Part model, mm, in its own coordinate system. A direction names the side the tool comes from. Round coordinates to 2 decimals unless told otherwise and drop trailing zeros. Write each loop counter-clockwise with the first axis right and the second up, starting at its lowest first coordinate (ties: lowest second). Pieces come first, ordered by that corner, then holes.
1) Saw through at C-C on x = 7. Write the cut outline in (y, z), and give its area (3 significant figures).
2) Saw through at D-D on y = 18.25. Write the cut outline in (x, z), and give its area (3 significant figures).
3) Saw through at A-A on y = 8. Write the cut outline in (x, z), and give its area (3 significant figures).
4) Drill centre lines: L1, parallel to Y at x = 39.5, z = 1; L2, parallel to X at y = 14.5, z = 4; L3, parallel to X at y = 13.75, z = 1.25. Where is each one in solid material? Low to high.
5) Which spindle directions (+Z, -Z, +X, -X, +Y, -Y) get a long thin tool onto all of the face, cutting with end or side? Do faces 1 (the flat face through (37.795, 10, 2)), 2 (the flat face through (47, 5, 8)), 3 (the flat face through (4, 5, 6)). Say none if no direction does.
6) Saw through at B-B on z = 6.5. Write the cut outline in (x, y).
7) Flat gauge pins, fed straight in: pin 1 (10 mm diameter, centred on x = 40.5, y = 6, fed in from +Z); pin 2 (2.5 mm diameter, centred on x = 4, z = 11.5, fed in from +Y); pin 3 (1 mm diameter, centred on x = 29.5, y = 5, fed in from +Z). Where does each tip first touch, or does it go through?
8) Pull direction X, two halves, no side cores. Call faces 4 (the cylindrical face through (16.04, 6.2, 2.54)), 5 (the cylindrical face through (10.69, 6.14, 2.54)), 6 (the flat face through (25, 0, 4)): +X half, -X half, draft (parallel to the pull), parting line (faces both ways), or undercut.
```python
from build123d import *

# Parameters (mm, degrees)
SKETCH1_R           = 8.106403635
SKETCH1_R_2         = 8.1
BOSS_EXTRUDE2_DEPTH = 5
FILLET1_R           = 4
SKETCH3_W           = 5.205268412
SKETCH3_H           = 16.38085221
BOSS_EXTRUDE3_DEPTH = 5
SKETCH2_R           = 1.575419973
CUT_EXTRUDE1_DEPTH  = 5


with BuildPart() as part:
    # Sketch1 → Boss-Extrude2 (new body)
    with BuildSketch(Plane.XY):
        with BuildLine():
            Line((0, 0), (50, 0))
            Line((50, 0), (50, 5))
            Line((50, 5), (40.794731588, 5))
            Line((40.794731588, 5), (40.794731588, 10.6))
            ThreePointArc((40.794731588, 10.6), (39.294731588, 29.859964052), (37.794731588, 10.6))
            Line((37.794731588, 10.6), (37.794731588, 5))
            Line((37.794731588, 5), (14.894731588, 5))
            Line((14.894731588, 5), (14.894731588, 10.6))
            ThreePointArc((14.894731588, 10.6), (13.394731588, 29.802927968), (11.894731588, 10.6))
            Line((11.894731588, 10.6), (11.894731588, 5))
            Line((11.894731588, 5), (0, 5))
            Line((0, 5), (0, 0))
        make_face()
        with Locations((13.394731588, 19.909096331)):
            Circle(SKETCH1_R, mode=Mode.SUBTRACT)
        with Locations((39.294731588, 19.909096331)):
            Circle(SKETCH1_R_2, mode=Mode.SUBTRACT)
    extrude(amount=BOSS_EXTRUDE2_DEPTH)

    # Fillet1
    fillet1_edges = [part.edges().sort_by_distance(p)[0] for p in [
        (11.894731588, 5, 2.5),
        (14.894731588, 5, 2.5),
        (37.794731588, 5, 2.5),
        (40.794731588, 5, 2.5),
    ]]
    fillet(fillet1_edges, radius=FILLET1_R)

    # Sketch3 → Boss-Extrude3 (add)
    with BuildSketch(Plane(origin=(0, 5, 0), x_dir=(1, 0, 0), z_dir=(0, 1, 0))):
        Polygon((5.642760672, 0), (0, 0), (0, -16.416233716), (6.001314969, -16.410881412), align=None)
        with Locations((47.397365794, -8.190426105)):
            Rectangle(SKETCH3_W, SKETCH3_H)
    extrude(amount=-BOSS_EXTRUDE3_DEPTH)

    # Sketch2 → Cut-Extrude1 (cut)
    with BuildSketch(Plane(origin=(0, 5, 0), x_dir=(1, 0, 0), z_dir=(0, 1, 0))):
        with Locations(Location((2.276803949, -12.5, 0), (0, 0, 180))):
            Circle(SKETCH2_R)
        with Locations(Location((47.26704488, -12.5, 0), (0, 0, 180))):
            Circle(SKETCH2_R)
    extrude(amount=-CUT_EXTRUDE1_DEPTH, mode=Mode.SUBTRACT)


solid = part.part
```
Completed:
1. outline: (0, 0) - (5, 0) - (5, 5) - (0, 5) - close; (12.9, 0) - (14.93, 0) - (14.93, 5) - (12.9, 5) - close; (24.89, 0) - (27.38, 0) - (27.38, 5) - (24.89, 5) - close
1. area: 47.6 mm2
2. outline: (3.92, 0) - (5.46, 0) - (5.46, 5) - (3.92, 5) - close; (21.33, 0) - (22.87, 0) - (22.87, 5) - (21.33, 5) - close; (29.8, 0) - (31.37, 0) - (31.37, 5) - (29.8, 5) - close; (47.22, 0) - (48.79, 0) - (48.79, 5) - (47.22, 5) - close
2. area: 31.1 mm2
3. outline: (11.77, 0) - (15.02, 0) - (15.02, 5) - (11.77, 5) - close; (37.67, 0) - (40.92, 0) - (40.92, 5) - (37.67, 5) - close
3. area: 32.5 mm2
4. L1: y = 0 to 11.81, 28.01 to 29.86
4. L2: x = 5.55 to 7.36, 19.43 to 21.24, 31.44 to 33.27, 45.32 to 47.15
4. L3: x = 6.15 to 8.12, 18.67 to 20.64, 32.04 to 34.03, 44.56 to 46.55
5. face 1: +Z, -Z
5. face 2: +Z, -Z, +X
5. face 3: +Z, -Z, -X
6. outline: (0, 0) - (5.78, 0) - (5.78, 5) - (0, 5) - close; (44.79, 0) - (50, 0) - (50, 5) - (44.79, 5) - close
7. pin 1: stops at z = 16.38
7. pin 2: stops at y = 5
7. pin 3: stops at z = 5
8. face 4: undercut
8. face 5: -X half
8. face 6: draft
